The listing builds one solid part. Answer for the finished solid, in the listing's coordinates (mm). A direction names the side the tool comes from. Coordinates: 2 decimals unless noted, no trailing zeros. Write each loop counter-clockwise with the first axis right and the second up, starting at its lowest first coordinate (ties: lowest second). Pieces come first, ordered by that corner, then holes. Notation, with made-up numbers: M 52.25,13 L 80.25,13 A24 cw 80.25,37 Z; hole C -23.75,81 d4. An arc over 180 degrees is marked long. Answer as CSV lines item,"result". Start each with the question number.
Autodesk Inventor part; units mm, degrees
ref_plane "YZ Plane" through (0, 0, 0) normal (1, 0, 0) x (0, 1, 0)
ref_plane "XZ Plane" through (0, 0, 0) normal (0, 1, 0) x (-1, 0, 0)
ref_plane "XY Plane" through (0, 0, 0) normal (0, 0, 1) x (1, 0, 0)
sketch "Sketch1" plane through (0, 0, 0) normal (0, 0, 1) x (1, 0, 0)
  line L0 (-127.5, 15) -> (127.5, 15)
  line L1 (127.5, 15) -> (127.5, -15)
  line L2 (127.5, -15) -> (-127.5, -15)
  line L3 (-127.5, -15) -> (-127.5, 15)
  line L4 (-127.5, 15) -> (127.5, -15) construction
  line L5 (127.5, 15) -> (-127.5, -15) construction
  point P0 (0, 0)
  dimension "d0" = 255
  dimension "d1" = 30
extrude "Extrusion1" add sketch "Sketch1" along normal blind 5
sketch "Sketch2" plane through (0, 0, 5) normal (0, 0, 1) x (1, 0, 0)
  line L0 (-127.5, -15) -> (127.5, -15)
  line L1 (-110, -15) -> (-90, -15)
  line L2 (-90, -15) -> (-90, -20)
  line L3 (-90, -20) -> (-110, -20)
  line L4 (-110, -20) -> (-110, -15)
  line L5 (-60, -15) -> (-40, -15)
  line L6 (-40, -15) -> (-40, -20)
  line L7 (-40, -20) -> (-60, -20)
  line L8 (-60, -20) -> (-60, -15)
  line L9 (-10, -15) -> (10, -15)
  line L10 (10, -15) -> (10, -20)
  line L11 (10, -20) -> (-10, -20)
  line L12 (-10, -20) -> (-10, -15)
  line L13 (40, -15) -> (60, -15)
  line L14 (60, -15) -> (60, -20)
  line L15 (60, -20) -> (40, -20)
  line L16 (40, -20) -> (40, -15)
  line L17 (90, -15) -> (110, -15)
  line L18 (110, -15) -> (110, -20)
  line L19 (110, -20) -> (90, -20)
  line L20 (90, -20) -> (90, -15)
  point P0 (0, 0)
  point P1 (60, -15)
  point P2 (40, -15)
  point P3 (-90, -15)
  point P4 (-40, -15)
  point P5 (-60, -15)
  point P6 (10, -15)
  point P7 (-10, -15)
  point P8 (110, -15)
  point P9 (90, -15)
  dimension "d4" = 20
  dimension "d5" = 5
  dimension "d6" = 17.5
  dimension "d9" = 50
  dimension "d14" = 17.5
extrude "Extrusion2" add sketch "Sketch2" against normal blind 5
sketch "Sketch3" plane through (0, 0, 5) normal (0, 0, 1) x (1, 0, 0)
  line L0 (9.5, 10) -> (44.5, 10)
  line L1 (49.5, 5) -> (49.5, -5)
  line L2 (44.5, -10) -> (9.5, -10)
  line L3 (4.5, -5) -> (4.5, 5)
  line L4 (4.5, 10) -> (49.5, -10) construction
  line L5 (49.5, 10) -> (4.5, -10) construction
  line L6 (0, -10) -> (0, 0)
  line L7 (-9.5, 10) -> (-44.5, 10)
  line L8 (-49.5, 5) -> (-49.5, -5)
  line L9 (-44.5, -10) -> (-9.5, -10)
  line L10 (-4.5, -5) -> (-4.5, 5)
  line L11 (-4.5, 10) -> (-49.5, -10) construction
  line L12 (-49.5, 10) -> (-4.5, -10) construction
  arc A0 (49.5, 5) -> (44.5, 10) centre (44.5, 5) ccw
  arc A1 (44.5, -10) -> (49.5, -5) centre (44.5, -5) ccw
  arc A2 (4.5, -5) -> (9.5, -10) centre (9.5, -5) ccw
  arc A3 (9.5, 10) -> (4.5, 5) centre (9.5, 5) ccw
  arc A4 (-4.5, 5) -> (-9.5, 10) centre (-9.5, 5) ccw
  arc A5 (-9.5, -10) -> (-4.5, -5) centre (-9.5, -5) ccw
  arc A6 (-44.5, 10) -> (-49.5, 5) centre (-44.5, 5) ccw
  arc A7 (-49.5, -5) -> (-44.5, -10) centre (-44.5, -5) ccw
  point P0 (27, 0)
  point P1 (-27, 0)
  dimension "d17" = 45
  dimension "d18" = 20
  dimension "d19" = 27
  dimension "d22" = 5
extrude "Extrusion3" cut sketch "Sketch3" against normal blind 10
properties part number "Divisória-25cm Frontal"
1) The part is cut by section C-C (z = 1.3). Count the separate pieces of the cut face and the enclosed holes in it, then the cut area to 3 significant figures.
2) The part is cut by section B-B (y = -1). Determine the outline of the cut face in (x, z), then the cut area to 3 significant figures.
3) For a pull along X with two mould halves and no side action, classify faces 5 (the face through (-2, 15, 2)), 6 (the face through (-127.5, 0, 2)), 7 (the face through (4.5, 0, 3)) as +X half, -X half, draft (parallel to the pull), parting line (faces both ways), or undercut.
4) The part is cut by section D-D (x = -79.5). Determine the outline of the cut face in (y, z).
5) The part is cut by section A-A (x = -16.5). Determine the outline of the cut face in (y, z), then the cut area to 3 significant figures.
6) Find the intervals of material crossed by line 1 (X direction, y = -18, z = 0.45); line 2 (X direction, y = -5, z = 3.2); line 3 (Y direction, x = -11, z = 2.35), in increasing order. Write a range as from..to.
7) Which of the six approach directions +Z, -Z, +X, -X, +Y, -Y give full straight-line access (tool end or side, diameter ignored) to faces 1 (the face through (-60, -18, 3)), 2 (the face through (119, -15, 2)), 3 (the face through (49.5, 0, 3)), 4 (the face through (-50, -20, 3))?
8) Each of these flat-tipped pins is pushed along its axis until it touches: P1, Ø2.5, axis at y = -16.5, z = 2, coming from the +X side; P2, Ø1.5, axis at x = -68.5, z = 3, coming from the -Y side; P3, Ø1.5, axis at y = -16.5, z = 2.5, coming from the -X side. Where does it stop, or does it pass through?
Completed:
1,separate pieces,"1"
1,enclosed holes,"2"
1,area,"6,390 mm²"
2,outline,"M -127.5,0 L -49.5,0 L -49.5,5 L -127.5,5 Z; M -4.5,0 L 4.5,0 L 4.5,5 L -4.5,5 Z; M 49.5,0 L 127.5,0 L 127.5,5 L 49.5,5 Z"
2,area,"825 mm²"
3,face 5,"draft"
3,face 6,"-X half"
3,face 7,"undercut"
4,outline,"M -15,0 L 15,0 L 15,5 L -15,5 Z"
5,outline,"M -15,0 L -10,0 L -10,5 L -15,5 Z; M 10,0 L 15,0 L 15,5 L 10,5 Z"
5,area,"50.0 mm²"
6,line 1,"-110..-90, -60..-40, -10..10, 40..60, 90..110"
6,line 2,"-127.5..-49.5, -4.5..4.5, 49.5..127.5"
6,line 3,"-15..-10, 10..15"
7,face 1,"+Z, -Z, -Y"
7,face 2,"+Z, -Z, +X, -Y"
7,face 3,"+Z, -Z"
7,face 4,"+Z, -Z, +X, -X, -Y"
8,P1,"x = 110"
8,P2,"y = -15"
8,P3,"x = -110"
